Design review of the part built by this model. Coordinates are the model's own, in mm. A direction names the side the tool comes from. Coordinates: 2 decimals unless noted, no trailing zeros. Write each loop counter-clockwise with the first axis right and the second up, starting at its lowest first coordinate (ties: lowest second). Pieces come first, ordered by that corner, then holes. Notation, with made-up numbers: (4.5, 57) - (29.5, 57) arc R16 ccw to (29.5, 80) - close; hole circle Ø7 at (-32, -13). An arc over 180 degrees is marked (long way). Answer as a JSON object with one key per item and string values.
```python
from build123d import *

# Parameters (mm, degrees)
F1_DEPTH    = 20
F2_W        = 35
F2_H        = 10
F3_DEPTH    = 5
F4_W        = 35
F4_H        = 10
F5_DEPTH    = 5
F7_DEPTH    = 25
F8_T1_DEPTH = 10
F9_R        = 3
F10_R       = 2
F11_R       = 2
F12_R       = 2
F14_DEPTH   = 15
F15_R       = 5.5
F16_DEPTH   = 2
F17_R       = 4.25
F18_DEPTH   = 110.5843026286
F19_R       = 1.8416313508
F20_DEPTH   = 10


# Not quite as in the source:
# - a fillet or chamfer that OpenCascade refuses, or shapes differently, is made with other operations: its cross-section is extruded or revolved along the edge and cut away or added


with BuildPart() as f1:
    # F0 (on Front) → F1 (new body)
    with BuildSketch(Plane.XZ):
        Polygon((48.965709947, 58.1432288134), (47.6666718414, 58.8932288134), (17.6666718414, 6.9317045863), (147.6666718414, 6.9317045863), (147.6666718414, 16.9317045863), (100.3461637657, 16.9317045863), (78.6067260984, 29.4829747755), (79.8567260984, 31.648038285), (62.5362180227, 41.648038285), (61.2862180227, 39.4829747755), (48.965709947, 46.5962234296), (43.965709947, 49.4829747755), align=None)
        with BuildLine():
            Line((45.06859563, 8.4317045863), (30.795836966, 16.6720856431))
            ThreePointArc((30.795836966, 16.6720856431), (28.4662078345, 19.7081174365), (28.965709947, 23.502212662))
            Line((28.965709947, 23.502212662), (40.715709947, 43.8538096509))
            ThreePointArc((40.715709947, 43.8538096509), (43.7517417405, 46.1834387824), (47.545836966, 45.6839366698))
            Line((47.545836966, 45.6839366698), (95.9083415922, 17.7618316052))
            ThreePointArc((95.9083415922, 17.7618316052), (98.2379707236, 12.1376093608), (93.4083415922, 8.4317045863))
            Line((93.4083415922, 8.4317045863), (45.06859563, 8.4317045863))
        make_face(mode=Mode.SUBTRACT)
    extrude(amount=F1_DEPTH)

    # F2 (on face) → F3 (cut)
    with BuildSketch(Plane.XZ.offset(20)):
        with Locations((130.1666718414, 11.9317045863)):
            Rectangle(F2_W, F2_H)
    extrude(amount=-F3_DEPTH, mode=Mode.SUBTRACT)

    # F4 (on face) → F5 (cut)
    with BuildSketch(Plane(origin=(0, 0, 0), x_dir=(-1, 0, 0), z_dir=(0, 1, 0))):
        with Locations((-130.1666718414, 11.9317045863)):
            Rectangle(F4_W, F4_H)
    extrude(amount=-F5_DEPTH, mode=Mode.SUBTRACT)

    # F6 (on face) → F7 (cut)
    with BuildSketch(Plane.XY.offset(16.9317045863)):
        with BuildLine():
            Line((147.6666718414, -7.0000102813), (130.6745260024, -7.0000102813))
            ThreePointArc((130.6745260024, -7.0000102813), (130.6666718414, -7), (130.6588176804, -7.0000102813))
            ThreePointArc((130.6588176804, -7.0000102813), (127.6666744117, -10.0039270839), (130.6666718414, -13))
            Line((130.6666718414, -13), (147.6666718414, -13))
            Line((147.6666718414, -13), (147.6666718414, -7.0000102813))
        make_face()
    extrude(amount=-F7_DEPTH, mode=Mode.SUBTRACT)

    # F8: fillet of radius 3 on 1 edges, made by hand

    # F8_s2 → F8_t1 (join)
    with BuildSketch(Plane.XY.offset(6.9317045863)):
        with BuildLine():
            add(Edge.make_bspline(
                [(112.6666718414, -18), (112.6666718414, -15), (115.6666718414, -15)],
                knots=[0, 0, 0, 1, 1, 1], degree=2, weights=[1, 1, 1]))
            Line((115.6666718414, -15), (112.6666718414, -15))
            Line((112.6666718414, -15), (112.6666718414, -18))
        make_face()
    extrude(amount=F8_T1_DEPTH)

    # F9
    f9_edges = [f1.edges().sort_by_distance(p)[0] for p in [
        (112.666672, -5, 11.931705),
    ]]
    fillet(f9_edges, radius=F9_R)

    # F10
    f10_edges = [f1.edges().sort_by_distance(p)[0] for p in [
        (78.606726, -10, 29.482975),
    ]]
    fillet(f10_edges, radius=F10_R)

    # F11
    f11_edges = [f1.edges().sort_by_distance(p)[0] for p in [
        (61.286218, -10, 39.482975),
    ]]
    fillet(f11_edges, radius=F11_R)

    # F12
    f12_edges = [f1.edges().sort_by_distance(p)[0] for p in [
        (43.96571, -10, 49.482975),
    ]]
    fillet(f12_edges, radius=F12_R)

    # F13 (on face) → F14 (cut)
    with BuildSketch(Plane(origin=(33.668184092, 0, 58.3150054459), x_dir=(0.8660254038, 0, -0.5), z_dir=(0.5, 0, 0.8660254038))):
        with BuildLine():
            Line((46.8339343218, -6), (39.8339343218, -6))
            ThreePointArc((39.8339343218, -6), (35.8339343218, -10), (39.8339343218, -14))
            Line((39.8339343218, -14), (46.8339343218, -14))
            ThreePointArc((46.8339343218, -14), (50.8339343218, -10), (46.8339343218, -6))
        make_face()
    extrude(amount=-F14_DEPTH, mode=Mode.SUBTRACT)

    # F15 (on face) → F16 (cut)
    with BuildSketch(Plane(origin=(10.2484877494, 0, -5.9169671609), x_dir=(0, -1, 0), z_dir=(-0.8660254038, 0, 0.5))):
        with Locations((10, 22.3363681839)):
            Circle(F15_R)
    extrude(amount=-F16_DEPTH, mode=Mode.SUBTRACT)

    # F17 (on face) → F18 (cut, through all)
    with BuildSketch(Plane(origin=(11.980538557, 0, -6.9169671609), x_dir=(0, -1, 0), z_dir=(-0.8660254038, 0, 0.5))):
        with Locations((10, 22.3363681839)):
            Circle(F17_R)
    extrude(amount=-F18_DEPTH, mode=Mode.SUBTRACT)

    # F19 (on face) → F20 (cut)
    with BuildSketch(Plane(origin=(10.2484877494, 0, -5.9169671609), x_dir=(0, -1, 0), z_dir=(-0.8660254038, 0, 0.5))):
        with Locations((15, 53.8363681839)):
            Circle(F19_R)
        with Locations((5, 53.8363681839)):
            Circle(F19_R)
        with Locations((5, 46.8363681839)):
            Circle(F19_R)
        with Locations((15, 46.8363681839)):
            Circle(F19_R)
        with Locations((15, 39.8363681839)):
            Circle(F19_R)
        with Locations((5, 39.8363681839)):
            Circle(F19_R)
    extrude(amount=-F20_DEPTH, mode=Mode.SUBTRACT)


solid = f1.part
```
(1) For pin 1 (8 mm diameter, centred on x = 137.5, z = 10.5, fed in from +Y); pin 2 (1.5 mm diameter, centred on y = -6, z = 19.5, fed in from +X); pin 3 (12 mm diameter, centred on y = -3.5, z = 18.5, fed in from -X); pin 4 (10 mm diameter, centred on x = 43, z = 42.5, fed in from -Y), all flat-tipped, find the tip position at first contact; note any pin that passes through.
Solved:
{"pin 1": "stops at y = -5", "pin 2": "stops at x = 97.2", "pin 3": "stops at x = 20.88", "pin 4": "stops at y = -20"}
(2) The part is to be moulded in two halves that separate along Z. For faces 1 (the face through (61, 0, 8)), 2 (the face through (63.716, -9.912, 38.69)), 3 (the face through (82, -10, 6.932)), say which applies: pulls with the +Z half, pulls with the -Z half, needs draft (parallel to the pull), parting line crosses it, or undercut.
Solved:
{"face 1": "needs draft", "face 2": "undercut", "face 3": "pulls with the -Z half"}
(3) Take a section at B-B, the plane x = 119. Write out the cut boundary in (y, z), and give its area (3 significant figures).
Solved:
{"outline": "(-15, 6.93) - (-5, 6.93) - (-5, 16.93) - (-15, 16.93) - close", "area": "100 mm^2"}
(4) To check wall thickness, follow line 1 (Y direction, x = 35, z = 35); line 2 (Z direction, x = 70, y = -14.75); line 3 (X direction, y = -17.25, z = 17.5). State the ranges of each line that lie inside material, in increasing order. Write a range as from..to.
Solved:
{"line 1": "y = -20..-16.56, -13.44..-6.56, -3.44..0", "line 2": "z = 6.93..8.43, 32.72..37.34", "line 3": "x = 23.77..29.73, 96.32..99.36"}
(5) Tool access review of faces 4 (the face through (71.389, -5.416, 31.918)), 5 (the face through (20.92, -9.97, 8.57)), 6 (the face through (76.705, -10.088, 31.191)), 7 (the face through (118, -10, 16.932)), 8 (the face through (139, -13, 12)): name each direction out of +Z, -Z, +X, -X, +Y, -Y from which nothing blocks a thin tool from reaching the whole face with its end or side.
Solved:
{"face 4": "+Y, -Y", "face 5": "none", "face 6": "+Z", "face 7": "+Z, +X, +Y, -Y", "face 8": "+Z, -Z, +X"}
